Geometry: final body of the model. Coordinates: model frame, mm. A direction names the side the tool comes from. Give positions to 0.01 mm unless a question says otherwise; leave off trailing zeros. Write each loop counter-clockwise with the first axis right and the second up, starting at its lowest first coordinate (ties: lowest second). Pieces come first, ordered by that corner, then holes. Notation, with made-up numbers: (-6.75, 54) -> (47.25, 54) arc R25 ccw to (47.25, 92) -> close; hole circle Ø8 at (89, -30.5). An arc over 180 degrees is marked (long way). Use CSV: the item, a comma, the result in double quotes. Start each with the question number.
1) Material intervals for line 1 (X direction, y = 1.5, z = -0.5); line 2 (Z direction, x = -2.5, y = -3); line 3 (X direction, y = 1.75, z = -0.75), sorted ascending. Write a range as [from, to].
2) Section A-A (z = -0.75). Output: boundary loops of the cut face in (x, y) (3 decimals), plus the area to 3 significant figures.
3) Contact query for flat-ended pins moving along their axis: P1, Ø1, axis at x = -3.5, y = -3.5, coming from the +Z side; P2, Ø1.3, axis at y = 0.5, z = 1.5, coming from the -X side; P3, Ø0.8, axis at x = 0, y = 0.5, coming from the +Z side. Output: stop coordinate, or through.
4) Set-up query: faces 5 (the face through (-0.5, 0, 1)), 6 (the face through (0, 0, 3)), 7 (the face through (0, 0, -1.5)), 8 (the face through (1, -4, 0.5)). Return all of +Z, -Z, +X, -X, +Y, -Y with unobstructed straight access to the full face (end or side cutting, diameter ignored); none if empty.
5) Section C-C (x = 4). Output: boundary loops of the cut face in (y, z).
6) Section B-B (y = 0). Count the separate pieces of the cut face and the enclosed holes in it, plus the area to 3 significant figures.
7) Draft query along Y for faces 1 (the face through (1.15, 2.22, 1.59)), 2 (the face through (1, -4, 1.5)), 3 (the face through (0.5, 0, 1)), 4 (the face through (-0.818, 3.685, 2.116)). Return one class per face: pulls with the +Y half, pulls with the -Y half, needs draft (parallel to the pull), parting line crosses it, or undercut.
Autodesk Fusion 360 part; units mm, degrees
sketch "Sketch1" plane through (0, 0, 0) normal (0, 0, 1) x (1, 0, 0)
  circle A0 centre (0, 0) radius 3.775
  circle A1 centre (0, 0) radius 1.5
  dimension "d1" = 7.55
  dimension "d2" = 3
extrude "Extrude1" add sketch "Sketch1" along normal blind 5 makes body 1
fillet "Fillet1" radius 2.25 1 edges at (-3.5195, -1.3651, 5) on bodies 1
sketch "Sketch2" plane through (0, 0, 0) normal (0, 0, -1) x (1, 0, 0)
  circle A0 centre (0, 0) radius 1.5
  circle A1 centre (0, 0) radius 3.775
  circle A2 centre (0, 0) radius 2
  dimension "d7" = 4
extrude "Extrude2" cut sketch "Sketch2" against normal blind 13.5 contours A2 bodies 1
extrude "Extrude3" cut 1 faces at (3.1618, -0.2869, 0) along direction (0, 0, 1) blind 1.5 on bodies 1 bodies 1
sketch "Sketch3" plane through (0, 0, 1.5) normal (0, 0, -1) x (1, 0, 0)
  circle A0 centre (0, 0) radius 2
  circle A1 centre (0, 0) radius 3.775
  circle A2 centre (0, 0) radius 5
  dimension "d12" = 10
extrude "Extrude4" add sketch "Sketch3" along normal blind 1 separate body contours A2 makes body 2
extrude "Extrude5" add 1 faces at (3.1618, -0.2869, 1.5) along direction (0, 0, -1) blind 3 on bodies 1 bodies 1 2
sketch "Sketch4" plane through (0, 0, -1.5) normal (0, 0, -1) x (1, 0, 0)
  circle A0 centre (0, 0) radius 2
  circle A1 centre (0, 0) radius 3.775
  circle A2 centre (0, 0) radius 2.5
  dimension "d17" = 5
extrude "Extrude6" cut sketch "Sketch4" against normal blind 12.5 contours A2 bodies 1
sketch "Sketch5" plane through (0, 0, -1.5) normal (0, 0, -1) x (1, 0, 0)
  circle A0 centre (0, 0) radius 2.5
  circle A1 centre (0, 0) radius 3.775
  line L0 (0, 3.5) -> (0, -3.5) construction
  line L1 (0.5, 3.5) -> (0.5, -3.5)
  line L2 (-0.5, 3.5) -> (-0.5, -3.5)
  dimension "d20" = -0.5
  dimension "d21" = 0.5
extrude "Extrude7" add sketch "Sketch5" against normal blind 4.5 contours A0 L1 L2 bodies 1
Answers follow:
1,line 1,"x = [-3.46, -2], [-0.5, 0.5], [2, 3.46]"
1,line 2,"z = [0.5, 1.5]"
1,line 3,"x = [-3.34, -1.79], [-0.5, 0.5], [1.79, 3.34]"
2,outline,"circle Ø7.55 at (0, 0); hole (-0.5, -2.449) -> (-0.5, 2.449) arc R2.5 ccw to start; hole (0.5, -2.449) arc R2.5 ccw to (0.5, 2.449) -> close"
2,area,"30.1 mm^2"
3,P1,"stops at z = 1.5"
3,P2,"stops at x = -5"
3,P3,"stops at z = 3"
4,face 5,"+Z, -Z"
4,face 6,"+Z"
4,face 7,"-Z, +X, -X, +Y, -Y"
4,face 8,"-Z"
5,outline,"(-3, 0.5) -> (3, 0.5) -> (3, 1.5) -> (-3, 1.5) -> close"
6,separate pieces,"3"
6,enclosed holes,"0"
6,area,"21.5 mm^2"
7,face 1,"undercut"
7,face 2,"needs draft"
7,face 3,"undercut"
7,face 4,"parting line crosses it"
